Could you check a few things on this drawing? It's one solid part, dimensions in mm from its lowest x, y, z. A direction names the side the tool comes from. Round coordinates to 2 decimals unless told otherwise and drop trailing zeros. Write each loop counter-clockwise with the first axis right and the second up, starting at its lowest first coordinate (ties: lowest second). Pieces come first, ordered by that corner, then holes. Notation, with made-up numbers: (-33, 11.5) -> (1, 11.5) arc R27 ccw to (1, 31.5) -> close; hole circle Ø4 at (53, 0). An arc over 180 degrees is marked (long way). Answer in a Markdown table with one row per item. Add a question column.
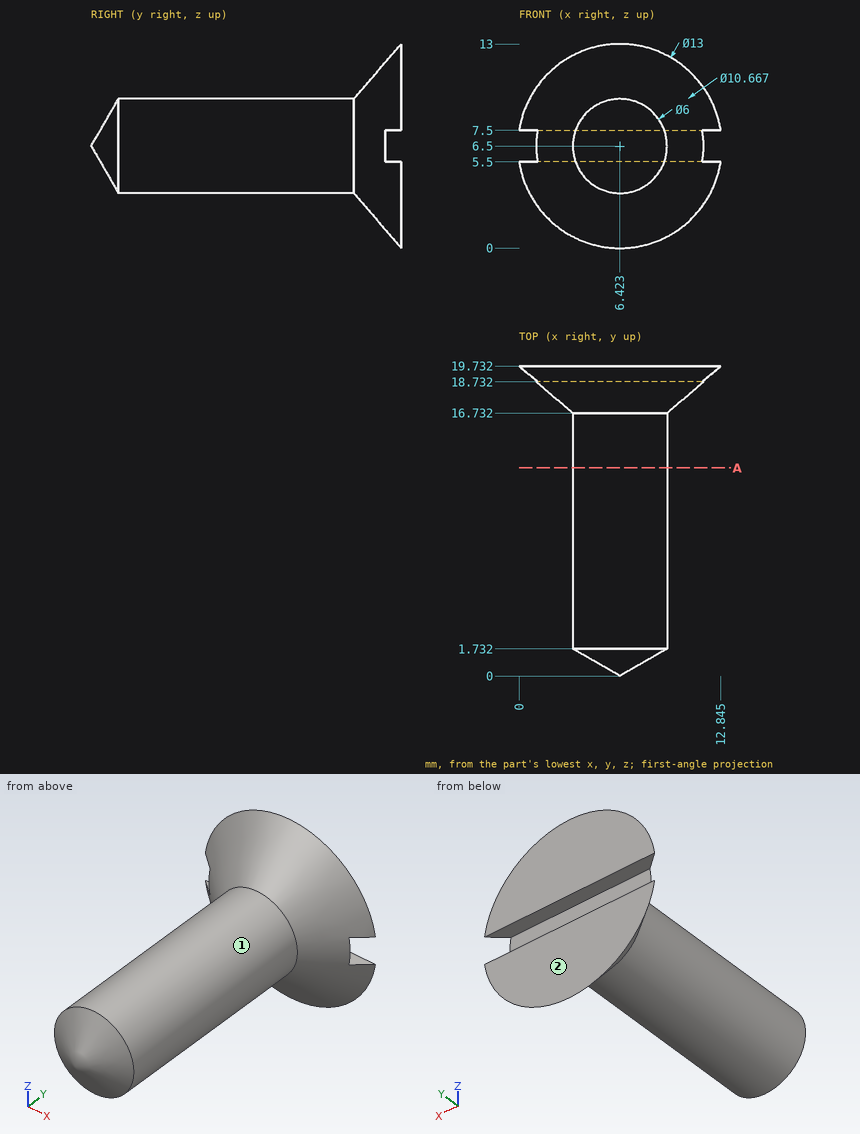
Item 1: On a 3-axis mill with a long thin cutter (end or side, diameter ignored), from which of +Z, -Z, +X, -X, +Y, -Y can I reach the whole of each face in a straight line? I mean the marked faces 1 and 2. Say none if no direction works.
Item 2: For P1, Ø1.5, axis at x = 5, y = 17, coming from the -Z side; P2, Ø1.5, axis at x = 4.5, y = 14, coming from the +Z side; P3, Ø2, axis at y = 12.5, z = 4.5, coming from the +X side; P4, Ø6, axis at x = 7.5, z = 6.5, coming from the -Y side, each with a flat end and sliding along its axis, tell me the tip position at first contact or that it passes through.
Item 3: I need wall thicknesses on line 1 along Y through (x, z) = (2.75, 11.5); line 2 along X through (y, z) = (18.5, 4.25) (1 decimal); line 3 along Y through (x, z) = (4.75, 8.5) (1 decimal). Which ranges of each line are inside material? Lowest first, please. Write a range as from..to.
Item 4: If we section it at A-A on y = 13.25: Please give me the cut outline in (x, z), then the cut area to 3 significant figures.
Results list:
| question | item | result |
|---|---|---|
| 1 | face 1 | -Y |
| 1 | face 2 | +Z, -Z, +X, -X, +Y |
| 2 | P1 | z = 2.53 |
| 2 | P2 | z = 9.26 |
| 2 | P3 | x = 9.25 |
| 2 | P4 | y = 0 |
| 3 | line 1 | 19.48..19.73 |
| 3 | line 2 | 1.9..11 |
| 3 | line 3 | 1.5..19.7 |
| 4 | outline | circle Ø6 at (6.42, 6.5) |
| 4 | area | 28.3 mm² |
